```python
from build123d import *

# Parameters (mm, degrees)
SKETCH_1_R      = 1.5
EXTRUDE_1_DEPTH = 4


with BuildPart() as part:
    # 草图1 → 凸台-拉伸1 (new body)
    with BuildSketch(Plane.XY):
        Polygon((-7, 7), (65.12, 7), (65.12, -15), (43.12, -15), (43.12, -93.617838822), (29.06, -210), (15, -93.617838822), (15, -13.617838822), (-7, -13.617838822), align=None)
        Circle(SKETCH_1_R, mode=Mode.SUBTRACT)
        with Locations((58.12, 0)):
            Circle(SKETCH_1_R, mode=Mode.SUBTRACT)
    extrude(amount=EXTRUDE_1_DEPTH)


solid = part.part
```
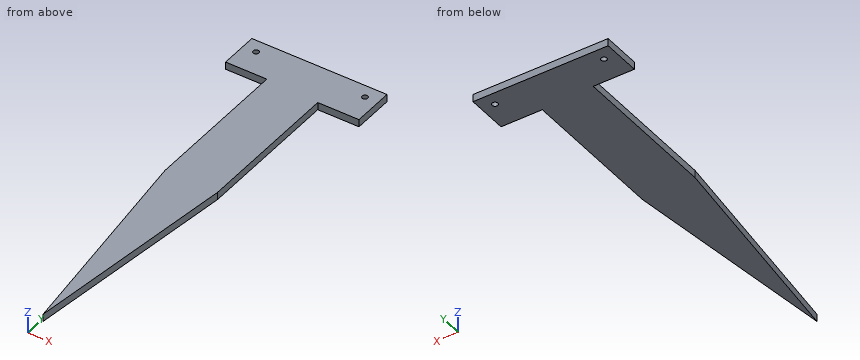
The listing builds one solid part. Answer for the finished solid, in the listing's coordinates (mm). Round coordinates to 2 decimals unless told otherwise and drop trailing zeros. Loops run counter-clockwise (first coordinate to the right, second up) from the corner with the lowest first, then second, coordinate; pieces in that order, holes last.
1) A cutting plane is placed at A-A on z = 0.9. Determine the outline of the cut face in (x, y).
Outcome:
outline: (-7, -13.62) - (15, -13.62) - (15, -93.62) - (29.06, -210) - (43.12, -93.62) - (43.12, -15) - (65.12, -15) - (65.12, 7) - (-7, 7) - close; hole circle Ø3 at (0, 0); hole circle Ø3 at (58.12, 0)
2) A cutting plane is placed at B-B on x = 11. Determine the outline of the cut face in (y, z).
Outcome:
outline: (-13.62, 0) - (7, 0) - (7, 4) - (-13.62, 4) - close
3) A cutting plane is placed at C-C on y = -178. Determine the outline of the cut face in (x, z), plus the area to 3 significant figures.
Outcome:
outline: (25.19, 0) - (32.93, 0) - (32.93, 4) - (25.19, 4) - close
area: 30.9 mm2
4) Consider line 1 (Y direction, x = 58.12, z = 3); line 2 (Y direction, x = 0, z = 1.15); line 3 (Y direction, x = 14, z = 3.8). Determine where each line is inside the solid, lowest interval first.
Outcome:
line 1: y = -15 to -1.5, 1.5 to 7
line 2: y = -13.62 to -1.5, 1.5 to 7
line 3: y = -13.62 to 7
5) Given P1, Ø4, axis at x = 0, y = 0, coming from the +Z side; P2, Ø1.2, axis at y = -54.5, z = 1, coming from the +X side; P3, Ø1.2, axis at x = 5.5, z = 2, coming from the -Y side; P4, Ø1.8, axis at x = 58.12, y = 0, coming from the -Z side, each flat-ended and moving along its own axis, determine where each tip first touches the part or whether it passes through.
Outcome:
P1: stops at z = 4
P2: stops at x = 43.12
P3: stops at y = -13.62
P4: passes through
